Answer from the drawing. Dimensions are ordinates in mm from the lowest x, y and z of the part. A direction names the side the tool comes from. Round coordinates to 2 decimals unless told otherwise and drop trailing zeros. Loops run counter-clockwise (first coordinate to the right, second up) from the corner with the lowest first, then second, coordinate; pieces in that order, holes last. Notation, with made-up numbers: M -1.5,2.25 L 22.5,2.25 A7 cw 22.5,6.25 Z; hole C 30.25,-37.75 d4. An arc over 180 degrees is marked long. Write each question's results on one line, items separated by ' | '.
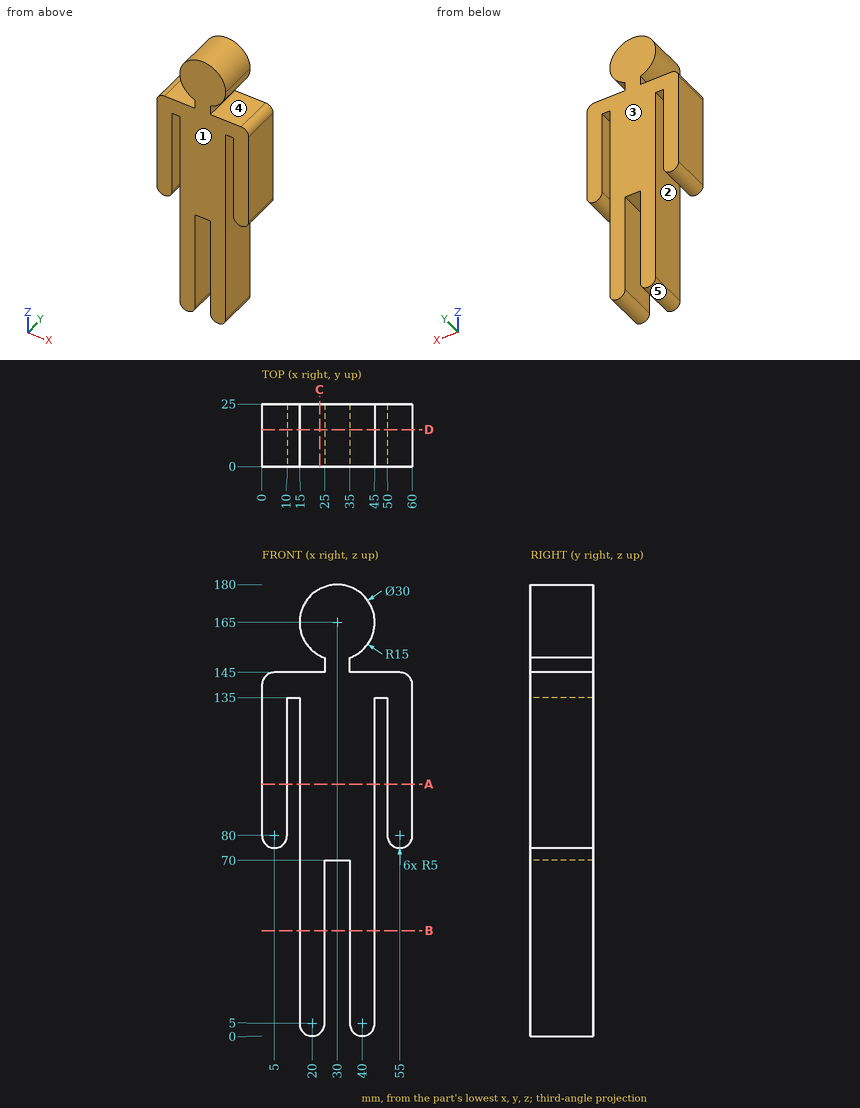
1. Given P1, Ø1, axis at x = 28, y = 18, coming from the -Z side; P2, Ø12.5, axis at y = 13, z = 21.5, coming from the -X side; P3, Ø2.5, axis at x = 13.5, y = 8.5, coming from the -Z side, each flat-ended and moving along its own axis, determine where each tip first touches the part or whether it passes through.
Completed:
P1: stops at z = 70 | P2: stops at x = 15 | P3: stops at z = 135
2. Find section D-D, the plane y = 14.75. Give the vertices of the cut face in (x, z), then the cut area to 3 significant figures.
Completed:
outline: M 0,80 A5 ccw 10,80 L 10,135 L 15,135 L 15,5 A5 ccw 25,5 L 25,70 L 35,70 L 35,5 A5 ccw 45,5 L 45,135 L 50,135 L 50,80 A5 ccw 60,80 L 60,140 A5 ccw 55,145 L 35,145 L 35,150.86 A15 ccw long 25,150.86 L 25,145 L 5,145 A5 ccw 0,140 Z | area: 5,860 mm2
3. Which of the six approach directions +Z, -Z, +X, -X, +Y, -Y give full straight-line access (tool end or side, diameter ignored) to the marked faces 1 and 2?
Completed:
face 1: +Z, -Z, +X, -X, -Y | face 2: -Z, +Y, -Y
4. Find section A-A, the plane z = 100.5. Give the vertices of the cut face in (x, y).
Completed:
outline: M 0,0 L 10,0 L 10,25 L 0,25 Z; M 15,0 L 45,0 L 45,25 L 15,25 Z; M 50,0 L 60,0 L 60,25 L 50,25 Z
5. Find section B-B, the plane z = 42. Give the vertices of the cut face in (x, y), then the cut area to 3 significant figures.
Completed:
outline: M 15,0 L 25,0 L 25,25 L 15,25 Z; M 35,0 L 45,0 L 45,25 L 35,25 Z | area: 500 mm2
6. Find the intervals of material crossed by L1, parallel to X at y = 12.75, z = 81; L2, parallel to X at y = 23.5, z = 149; L3, parallel to Z at x = 29.5, y = 1.75, in increasing order.
Completed:
L1: x = 0 to 10, 15 to 45, 50 to 60 | L2: x = 25 to 35 | L3: z = 70 to 179.99
7. Determine the mould class of the marked faces 3, 4 and 5 for opening direction Z: released by +Z, released by -Z, zero draft, split by the parting line, or undercut.
Completed:
face 3: zero draft | face 4: undercut | face 5: released by -Z
8. Find section C-C, the plane x = 23. Give the vertices of the cut face in (y, z), then the cut area to 3 significant figures.
Completed:
outline: M 0,1 L 25,1 L 25,145 L 0,145 Z; M 0,151.73 L 25,151.73 L 25,178.27 L 0,178.27 Z | area: 4,260 mm2
